Could you check a few things on this model? Use its own coordinates, in mm. A direction names the side the tool comes from. Round coordinates to 2 decimals unless told otherwise and drop trailing zeros. Write each loop counter-clockwise with the first axis right and the second up, starting at its lowest first coordinate (ties: lowest second). Pieces come first, ordered by that corner, then holes. Notation, with made-up numbers: (17, 21.25) -> (30, 21.25) arc R25 cw to (30, 48.25) -> close; hole circle Ø3 at (58, 19.5). An arc over 180 degrees is marked (long way). Return JSON: item names as keys, results as strings.
from build123d import *

# Parameters (mm, degrees)
F1_DEPTH = 50.8


with BuildPart() as f1:
    # F0 (on Front) → F1 (new body)
    with BuildSketch(Plane.XZ):
        with BuildLine():
            Line((0, 37.338), (0, 0))
            Line((0, 0), (37.338, 0))
            ThreePointArc((37.338, 0), (37.876815, 0.223185), (38.1, 0.762))
            Line((38.1, 0.762), (38.1, 2.413))
            ThreePointArc((38.1, 2.413), (37.876815, 2.951815), (37.338, 3.175))
            Line((37.338, 3.175), (6.35, 3.175))
            ThreePointArc((6.35, 3.175), (4.104936, 4.104936), (3.175, 6.35))
            Line((3.175, 6.35), (3.175, 37.338))
            ThreePointArc((3.175, 37.338), (2.951815, 37.876815), (2.413, 38.1))
            Line((2.413, 38.1), (0.762, 38.1))
            ThreePointArc((0.762, 38.1), (0.223185, 37.876815), (0, 37.338))
        make_face()
    extrude(amount=F1_DEPTH)


solid = f1.part
1) Will these pins go through, and if not, where does the flat tip stop? pin 1 Ø10 at (x, z) = (26.5, 11.5) entering from -Y; pin 2 Ø6 at (y, z) = (-18, 8.5) entering from +X; pin 3 Ø15.5 at (y, z) = (-14, 24.5) entering from +X (3 decimals); pin 4 Ø1 at (x, y) = (26, -16.5) entering from +Z (3 decimals).
Return value:
{"pin 1": "through", "pin 2": "x = 3.29", "pin 3": "x = 3.175", "pin 4": "z = 3.175"}
2) I want a section at B-B, the plane x = 22.5. Please give me the cut outline in (y, z) (3 decimals), and give its area (3 significant figures).
Return value:
{"outline": "(-50.8, 0) -> (0, 0) -> (0, 3.175) -> (-50.8, 3.175) -> close", "area": "161 mm²"}
3) I want a section at C-C, the plane z = 30. Please give me the cut outline in (x, y) (3 decimals).
Return value:
{"outline": "(0, -50.8) -> (3.175, -50.8) -> (3.175, 0) -> (0, 0) -> close"}
4) I want a section at A-A, the plane y = -45. Please give me the cut outline in (x, z) (3 decimals).
Return value:
{"outline": "(0, 0) -> (37.338, 0) arc R0.762 ccw to (38.1, 0.762) -> (38.1, 2.413) arc R0.762 ccw to (37.338, 3.175) -> (6.35, 3.175) arc R3.175 cw to (3.175, 6.35) -> (3.175, 37.338) arc R0.762 ccw to (2.413, 38.1) -> (0.762, 38.1) arc R0.762 ccw to (0, 37.338) -> close"}
5) If I drill on probe 1 along X at (y, z) = (-38.5, 24) (3 decimals), over which ranges is the centre line in solid material (lowest first)? Write a range as [from, to].
Return value:
{"probe 1": "[0, 3.175]"}
6) For faces 1 (the face through (0, -25, 19)), 2 (the face through (22, -25, 3.175)), which set-ups out of +Z, -Z, +X, -X, +Y, -Y let a thin tool reach every point of the face, with its end or its side?
Return value:
{"face 1": "+Z, -Z, -X, +Y, -Y", "face 2": "+Z, +X, +Y, -Y"}
